Source: CAD feature listing. Evaluate the final solid. Frame: model axes, mm. Face numbers are marked on the shaded views. A direction names the side the tool comes from. Coordinates: 2 decimals unless noted, no trailing zeros. Write each loop counter-clockwise with the first axis right and the second up, starting at its lowest first coordinate (ties: lowest second). Pieces come first, ordered by that corner, then holes. Notation, with made-up numbers: (-7.75, 8) - (15.25, 8) arc R21 ccw to (15.25, 42) - close; hole circle Ø8 at (7, -36.5). An arc over 180 degrees is marked (long way). One line per item, written item: value.
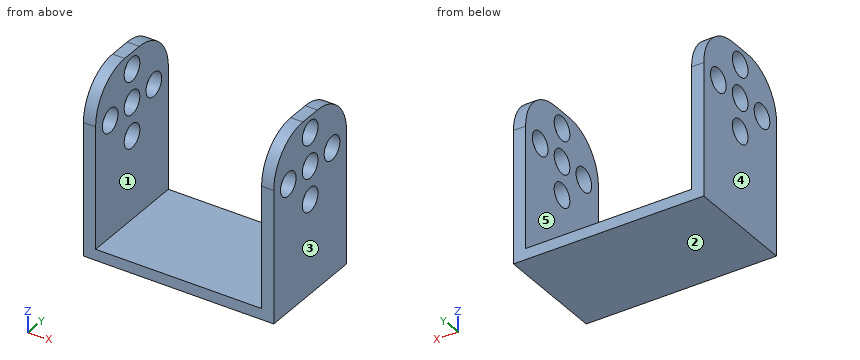
Autodesk Inventor part; units mm, degrees
ref_plane "YZ Plane" through (0, 0, 0) normal (1, 0, 0) x (0, 1, 0)
ref_plane "XZ Plane" through (0, 0, 0) normal (0, 1, 0) x (-1, 0, 0)
ref_plane "XY Plane" through (0, 0, 0) normal (0, 0, 1) x (1, 0, 0)
sketch "Esquisse1" plane through (0, 0, 0) normal (0, 0, 1) x (1, 0, 0)
  line L0 (0, 0) -> (34.4, 0)
  line L1 (34.4, 0) -> (34.4, 20)
  line L2 (34.4, 20) -> (0, 20)
  line L3 (0, 20) -> (0, 0)
  dimension "d0" = 34.4
  dimension "d1" = 20
extrude "Extrusion1" add sketch "Esquisse1" along normal blind 2
sketch "Esquisse2" plane through (0, 0, 2) normal (0, 0, 1) x (1, 0, 0)
  line L0 (0, 0) -> (34.4, 0)
  line L1 (34.4, 20) -> (0, 20)
  line L2 (0, 20) -> (0, 0)
  line L3 (0, 20) -> (2.2, 20)
  line L4 (2.2, 20) -> (2.2, 0)
  line L5 (2.2, 0) -> (0, 0)
  line L6 (0, 0) -> (0, 20)
  line L7 (17.2, 20) -> (17.2, 0) construction
  line L8 (34.4, 20) -> (32.2, 20)
  line L9 (32.2, 20) -> (32.2, 0)
  line L10 (32.2, 0) -> (34.4, 0)
  line L11 (34.4, 0) -> (34.4, 20)
  dimension "d4" = 2.2
extrude "Extrusion2" add sketch "Esquisse2" along normal blind 30 contours L2 L1 L4 L0 | L9 L1 L11 L0
sketch "Esquisse3" plane through (34.4, 0, 0) normal (1, 0, 0) x (0, 0, -1)
  line L0 (0, 0) -> (0, 20) construction
  line L1 (-32, 0) -> (-32, 20) construction
  line L2 (-32, 10) -> (0, 10) construction
  circle A0 centre (-23, 10) radius 2.15
  line L3 (-23, 10) -> (-23, 15.2246) construction
  circle A1 centre (-17, 10) radius 2.15
  circle A2 centre (-29, 10) radius 2.15
  circle A3 centre (-23, 10) radius 2.15
  circle A4 centre (-23, 16) radius 2.15
  circle A5 centre (-23, 4) radius 2.15
  circle A6 centre (-23, 10) radius 2.15
  dimension "d7" = 9
  dimension "d8" = 4.3
  dimension "d11" = 6
  dimension "d14" = 6
  dimension "d19" = 6
  dimension "d22" = 6
extrude "Extrusion3" cut sketch "Esquisse3" against normal through all
fillet "Congé1" radius 8 4 edges at (33.3, 20, 32) (1.1, 20, 32) (1.1, 0, 32) (33.3, 0, 32)
properties part number "U"
1) Section query A-A on z = 23. State how many separate pieces and enclosed holes the cut face has, then the cut area to 3 significant figures.
Values found:
separate pieces: 8
enclosed holes: 0
area: 31.2 mm2
2) Draft query along X for the marked faces 1, 2 and 3. Return one class per face: released by +X, released by -X, zero draft, split by the parting line, or undercut.
Values found:
face 1: undercut
face 2: zero draft
face 3: released by +X
3) Contact query for flat-ended pins moving along their axis: P1, Ø4, axis at y = 10, z = 29, coming from the +X side; P2, Ø6, axis at x = 14.5, y = 7.5, coming from the +Z side. Output: stop coordinate, or through.
Values found:
P1: through
P2: z = 2
4) Section query D-D on y = 14.75. Output: boundary loops of the cut face in (x, z), then the cut area to 3 significant figures.
Values found:
outline: (0, 0) - (34.4, 0) - (34.4, 21.25) - (32.2, 21.25) - (32.2, 2) - (2.2, 2) - (2.2, 21.25) - (0, 21.25) - close; (0, 24.75) - (2.2, 24.75) - (2.2, 31.51) - (0, 31.51) - close; (32.2, 24.75) - (34.4, 24.75) - (34.4, 31.51) - (32.2, 31.51) - close
area: 183 mm2
5) Section query C-C on z = 17. Output: boundary loops of the cut face in (x, y), then the cut area to 3 significant figures.
Values found:
outline: (0, 0) - (2.2, 0) - (2.2, 7.85) - (0, 7.85) - close; (0, 12.15) - (2.2, 12.15) - (2.2, 20) - (0, 20) - close; (32.2, 0) - (34.4, 0) - (34.4, 7.85) - (32.2, 7.85) - close; (32.2, 12.15) - (34.4, 12.15) - (34.4, 20) - (32.2, 20) - close
area: 69.1 mm2
6) Reachability of the marked faces 4 and 5 from +Z, -Z, +X, -X, +Y, -Y: full face, straight path, thin tool, end or side. Return the list, or none.
Values found:
face 4: +Z, -Z, -X, +Y, -Y
face 5: +Z, +Y, -Y
7) Material intervals for line 1 (Y direction, x = 33, z = 23); line 2 (X direction, y = 3.75, z = 12.5); line 3 (Y direction, x = 1, z = 17), sorted ascending.
Values found:
line 1: 0 to 1.85, 6.15 to 7.85, 12.15 to 13.85, 18.15 to 20
line 2: 0 to 2.2, 32.2 to 34.4
line 3: 0 to 7.85, 12.15 to 20
